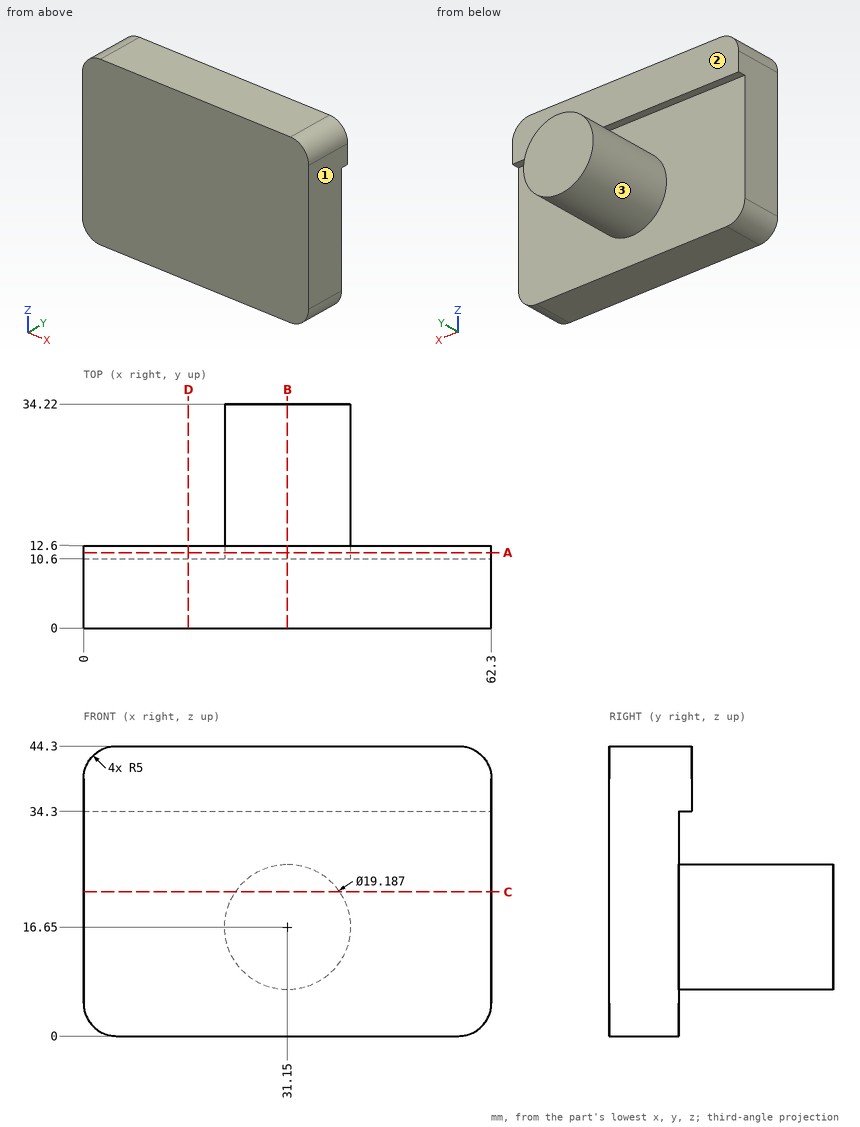
The drawing under review shows one solid part. Ordinate dimensions are in mm from its lowest x, y, z. A direction names the side the tool comes from. Coordinates: 2 decimals unless noted, no trailing zeros. Loops run counter-clockwise (first coordinate to the right, second up) from the corner with the lowest first, then second, coordinate; pieces in that order, holes last.
Item 1: Add section C-C (z = 22). Write out the cut boundary in (x, y), and give its area (3 significant figures).
Completed:
outline: (0, 0) - (62.3, 0) - (62.3, 10.6) - (39.11, 10.6) - (39.11, 34.22) - (23.19, 34.22) - (23.19, 10.6) - (0, 10.6) - close
area: 1,040 mm2
Item 2: Add section D-D (x = 16). Write out the cut boundary in (y, z).
Completed:
outline: (0, 0) - (10.6, 0) - (10.6, 34.3) - (12.6, 34.3) - (12.6, 44.3) - (0, 44.3) - close
Item 3: Clearance check with flat-ended pins moving along their axes: pin 1 (0.6 mm diameter, centred on x = 30, y = 12, fed in from -Z); pin 2 (11 mm diameter, centred on x = 36.5, z = 38.5, fed in from +Y); pin 3 (4 mm diameter, centred on x = 9.5, z = 24.5, fed in from +Y); pin 4 (5 mm diameter, centred on y = 17.5, z = 30.5, fed in from -X). State where each tip first meets the part, or that it passes through.
Completed:
pin 1: stops at z = 7.09
pin 2: stops at y = 12.6
pin 3: stops at y = 10.6
pin 4: passes through
Item 4: Add section B-B (x = 31.15). Write out the cut boundary in (y, z).
Completed:
outline: (0, 0) - (10.6, 0) - (10.6, 7.06) - (34.22, 7.06) - (34.22, 26.24) - (10.6, 26.24) - (10.6, 34.3) - (12.6, 34.3) - (12.6, 44.3) - (0, 44.3) - close
Item 5: Wall thickness on L1, parallel to Y at x = 13, z = 8.5; L2, parallel to Z at x = 52, y = 11.5; L3, parallel to Y at x = 22.5, z = 36.5: over which ranges is each line inside the solid? List them lowest first.
Completed:
L1: y = 0 to 10.6
L2: z = 34.3 to 44.3
L3: y = 0 to 12.6
Item 6: Add section A-A (y = 11.5). Write out the cut boundary in (x, z).
Completed:
outline: (0, 34.3) - (62.3, 34.3) - (62.3, 39.3) arc R5 ccw to (57.3, 44.3) - (5, 44.3) arc R5 ccw to (0, 39.3) - close; circle Ø19.19 at (31.15, 16.65)
Item 7: For the marked faces 1, 2 and 3, list the 3-axis set-ups (+Z, -Z, +X, -X, +Y, -Y) from which the entire face can be reached by the end or side of a thin tool; tool diameter is ignored.
Completed:
face 1: +Z, -Z, +X, +Y, -Y
face 2: +Z, +X, -X, +Y
face 3: +Y
